from build123d import *

# Parameters (mm, degrees)
SKETCH_1_W      = 6
SKETCH_1_H      = 6
EXTRUDE_1_DEPTH = 3
SKETCH_2_R      = 1
EXTRUDE_2_DEPTH = 4
SKETCH_3_R      = 1
EXTRUDE_3_DEPTH = 4
FILLET_1_R      = 0.1


with BuildPart() as part:
    # 草图1 → 凸台-拉伸1 (new body, symmetric)
    with BuildSketch(Plane.XY):
        Rectangle(SKETCH_1_W, SKETCH_1_H)
    extrude(amount=EXTRUDE_1_DEPTH, both=True)

    # 草图4 → 切除-旋转4 (revolve, cut)
    with BuildSketch(Plane(origin=(0, 0, 0), x_dir=(1, 0, 0), z_dir=(0, 1, 0))):
        with BuildLine():
            Line((0, -4.5), (0, -6.318562405))
            Line((0, -6.318562405), (-7, -6.318562405))
            Line((-7, -6.318562405), (-7, 6.288804718))
            Line((-7, 6.288804718), (0, 6.288804718))
            Line((0, 6.288804718), (0, 4.5))
            ThreePointArc((0, 4.5), (-4.5, 0), (0, -4.5))
        make_face()
    revolve(axis=Axis((0, 0, -4.5), (0, 0, 1)), mode=Mode.SUBTRACT)

    # 草图2 → 凸台-拉伸2 (add, symmetric)
    with BuildSketch(Plane.XY):
        Circle(SKETCH_2_R)
    extrude(amount=EXTRUDE_2_DEPTH, both=True)

    # 草图3 → 凸台-拉伸3 (add, symmetric)
    with BuildSketch(Plane(origin=(0, 0, 0), x_dir=(0, 0, -1), z_dir=(1, 0, 0))):
        Circle(SKETCH_3_R)
    extrude(amount=EXTRUDE_3_DEPTH, both=True)

    # 圆角1
    fillet_1_edges = [part.edges().sort_by_distance(p)[0] for p in [
        (-1, 0, -4),
        (-1, 0, 4),
        (-4, 0, 1),
        (4, 0, 1),
    ]]
    fillet(fillet_1_edges, radius=FILLET_1_R)


solid = part.part
Geometry check sheet. Reference: the model listing, model coordinates, mm. A direction names the side the tool comes from. Round coordinates to 2 decimals unless told otherwise and drop trailing zeros. Order: outer loops, then holes, each group sorted by start corner. A loop starts at its lowest first (then second) coordinate and runs counter-clockwise, first axis right, second up. Notation, with made-up numbers: M 62.5,77.25 L 87.5,77.25 A19 ccw 87.5,108.25 Z; hole C 26.25,2 d2. An arc over 180 degrees is marked long. Answer in a Markdown table with one row per item. Add a question column.
Item 1: Set-up check for faces 1 (the face through (3.456, -0.976, 0.217)), 2 (the face through (-3, -1, 1)), 3 (the face through (-0.217, -0.976, -3.444)), 4 (the face through (-0.217, -0.976, 3.456)): record each of +Z, -Z, +X, -X, +Y, -Y from which the full face is reachable in a straight line by a thin tool's end or side.
Item 2: Sectioned sample at A-A, the plane x = 0. Enter the section's corners in (y, z), plus the area to 3 significant figures.
Item 3: Sectioned sample at C-C, the plane y = 0. Enter the section's corners in (x, z).
Item 4: Depth check by flat-ended pin: pin 1 Ø2 at (x, y) = (-2.5, -1.5) entering from +Z; pin 2 Ø1 at (x, y) = (-1, -2.5) entering from -Z; pin 3 Ø1 at (y, z) = (-1, -2.5) entering from +X. Enter the tip coordinate at first touch or a pass-through.
Item 5: Sectioned sample at B-B, the plane z = 0. Enter the section's corners in (x, y), plus the area to 3 significant figures.
Item 6: Material ranges on L1, parallel to X at y = 0.7, z = -1.5; L2, parallel to Y at x = -2.75, z = 2.75, recorded low to high. Write a range as [from, to].
Item 7: Sectioned sample at D-D, the plane y = 1.95. Enter the section's corners in (x, z).
Filled in:
| question | item | result |
|---|---|---|
| 1 | face 1 | +X |
| 1 | face 2 | -X |
| 1 | face 3 | -Z |
| 1 | face 4 | +Z |
| 2 | outline | M -3,-3 L -1,-3 L -1,-3.9 A0.1 ccw -0.9,-4 L 0.9,-4 A0.1 ccw 1,-3.9 L 1,-3 L 3,-3 L 3,3 L 1,3 L 1,3.9 A0.1 ccw 0.9,4 L -0.9,4 A0.1 ccw -1,3.9 L -1,3 L -3,3 Z |
| 2 | area | 40.0 mm² |
| 3 | outline | M -4,-0.9 A0.1 ccw -3.9,-1 L -3,-1 L -3,-3 L -1,-3 L -1,-3.9 A0.1 ccw -0.9,-4 L 0.9,-4 A0.1 ccw 1,-3.9 L 1,-3 L 3,-3 L 3,-1 L 3.9,-1 A0.1 ccw 4,-0.9 L 4,0.9 A0.1 ccw 3.9,1 L 3,1 L 3,3 L 1,3 L 1,3.9 A0.1 ccw 0.9,4 L -0.9,4 A0.1 ccw -1,3.9 L -1,3 L -3,3 L -3,1 L -3.9,1 A0.1 ccw -4,0.9 Z |
| 4 | pin 1 | stops at z = 3 |
| 4 | pin 2 | stops at z = -3 |
| 4 | pin 3 | stops at x = 3 |
| 5 | outline | M -4,-0.9 A0.1 ccw -3.9,-1 L -3,-1 L -3,-3 L 3,-3 L 3,-1 L 3.9,-1 A0.1 ccw 4,-0.9 L 4,0.9 A0.1 ccw 3.9,1 L 3,1 L 3,3 L -3,3 L -3,1 L -3.9,1 A0.1 ccw -4,0.9 Z |
| 5 | area | 40.0 mm² |
| 6 | L1 | x = [-3, 3] |
| 6 | L2 | y = [-2.26, 2.26] |
| 7 | outline | M -3,-2.73 A4.06 ccw -2.73,-3 L 2.73,-3 A4.06 ccw 3,-2.73 L 3,2.73 A4.06 ccw 2.73,3 L -2.73,3 A4.06 ccw -3,2.73 Z |
